from build123d import *

# Parameters (mm, degrees)
S01_RETAINING_FLANGE_R                         = 6.25
F_01_RETAINING_FLANGE_DEPTH                    = 0.4
F_02_START                                     = 0.4
S02_INNER_RACE_AND_SEALED_ROLLING_ASSE_R       = 6.05
F_02_INNER_RACE_AND_SEALED_ROLLING_ASSEM_DEPTH = 11
F_03_START                                     = 11.4
S03_MOUNTING_THRUST_FACE_R                     = 6.25
F_03_MOUNTING_THRUST_FACE_DEPTH                = 0.6
F_04_START                                     = 12
S04_SIX_MILLIMETRE_STUD_WITH_FINAL_8_M_R       = 3
F_04_SIX_MILLIMETRE_STUD_WITH_FINAL_8_MM_DEPTH = 16
F_05_START                                     = -0.1
S05_ASSEMBLY_DRIVE_SLOT_W                      = 8.4
S05_ASSEMBLY_DRIVE_SLOT_H                      = 1.4
F_05_ASSEMBLY_DRIVE_SLOT_DEPTH                 = 0.7


with BuildPart() as part:
    # S01 - Retaining flange → 01 - Retaining flange (new body)
    with BuildSketch(Plane.XY):
        Circle(S01_RETAINING_FLANGE_R)
    extrude(amount=F_01_RETAINING_FLANGE_DEPTH)

    # S02 - Inner race and sealed rolling assembly envelope → 02 - Inner race and sealed rolling assembly envelope (add)
    with BuildSketch(Plane.XY.offset(F_02_START)):
        Circle(S02_INNER_RACE_AND_SEALED_ROLLING_ASSE_R)
    extrude(amount=F_02_INNER_RACE_AND_SEALED_ROLLING_ASSEM_DEPTH)

    # S03 - Mounting thrust face → 03 - Mounting thrust face (add)
    with BuildSketch(Plane.XY.offset(F_03_START)):
        Circle(S03_MOUNTING_THRUST_FACE_R)
    extrude(amount=F_03_MOUNTING_THRUST_FACE_DEPTH)

    # S04 - Six millimetre stud with final 8 mm M6 thread envelope → 04 - Six millimetre stud with final 8 mm M6 thread envelope (add)
    with BuildSketch(Plane.XY.offset(F_04_START)):
        Circle(S04_SIX_MILLIMETRE_STUD_WITH_FINAL_8_M_R)
    extrude(amount=F_04_SIX_MILLIMETRE_STUD_WITH_FINAL_8_MM_DEPTH)

    # S05 - Assembly drive slot → 05 - Assembly drive slot (cut)
    with BuildSketch(Plane.XY.offset(F_05_START)):
        Rectangle(S05_ASSEMBLY_DRIVE_SLOT_W, S05_ASSEMBLY_DRIVE_SLOT_H)
    extrude(amount=F_05_ASSEMBLY_DRIVE_SLOT_DEPTH, mode=Mode.SUBTRACT)


solid = part.part
Could you check a few things on this model? Use its own coordinates, in mm. A direction names the side the tool comes from. Round coordinates to 2 decimals unless told otherwise and drop trailing zeros. Write each loop counter-clockwise with the first axis right and the second up, starting at its lowest first coordinate (ties: lowest second). Pieces come first, ordered by that corner, then holes. Notation, with made-up numbers: (12, 61) - (69, 61) arc R31 cw to (69, 87) - close; hole circle Ø11 at (68.5, 40). An arc over 180 degrees is marked (long way). Use a Markdown table: item, result.
Q1. For faces 1 (the cylindrical face through (5.96, 1.88, 0.2)), 2 (the flat face through (-1, -3, 12)), which set-ups out of +Z, -Z, +X, -X, +Y, -Y let a thin tool reach every point of the face, with its end or its side?
Output values:
| item | result |
|---|---|
| face 1 | +Z, -Z |
| face 2 | +Z |
Q2. Please list where these lines run through material, in increasing order: L1, parallel to Z at x = 1.75, y = 5.75; L2, parallel to X at y = -0.25, z = 6.5; L3, parallel to Y at x = 2.75, z = 10.75.
Output values:
| item | result |
|---|---|
| L1 | 0 to 12 |
| L2 | -6.04 to 6.04 |
| L3 | -5.39 to 5.39 |
Q3. Thinking about a two-plate mould opening in Y: for faces 3 (the cylindrical face through (5.589, -2.317, 5.823)), 4 (the flat face through (0, -1, 0)), 5 (the flat face through (0, 0, 0.6)), which applies, released by +Y, released by -Y, zero draft, split by the parting line, or undercut?
Output values:
| item | result |
|---|---|
| face 3 | split by the parting line |
| face 4 | zero draft |
| face 5 | undercut |
Q4. I want a section at A-A (x = 0). List the corners of the cut face in (y, z) for me.
Output values:
| item | result |
|---|---|
| outline | (-6.25, 0) - (-0.7, 0) - (-0.7, 0.6) - (0.7, 0.6) - (0.7, 0) - (6.25, 0) - (6.25, 0.4) - (6.05, 0.4) - (6.05, 11.4) - (6.25, 11.4) - (6.25, 12) - (3, 12) - (3, 28) - (-3, 28) - (-3, 12) - (-6.25, 12) - (-6.25, 11.4) - (-6.05, 11.4) - (-6.05, 0.4) - (-6.25, 0.4) - close |
Q5. I want a section at C-C (z = 6.25). List the corners of the cut face in (x, y) for me, plus the area to 3 significant figures.
Output values:
| item | result |
|---|---|
| outline | circle Ø12.1 at (0, 0) |
| area | 115 mm2 |
Q6. I want a section at B-B (y = 0). List the corners of the cut face in (x, z) for me, plus the area to 3 significant figures.
Output values:
| item | result |
|---|---|
| outline | (-6.25, 0) - (-4.2, 0) - (-4.2, 0.6) - (4.2, 0.6) - (4.2, 0) - (6.25, 0) - (6.25, 0.4) - (6.05, 0.4) - (6.05, 11.4) - (6.25, 11.4) - (6.25, 12) - (3, 12) - (3, 28) - (-3, 28) - (-3, 12) - (-6.25, 12) - (-6.25, 11.4) - (-6.05, 11.4) - (-6.05, 0.4) - (-6.25, 0.4) - close |
| area | 237 mm2 |
Q7. For pin 1 (2 mm diameter, centred on y = -1.5, z = 9, fed in from +X); pin 2 (0.5 mm diameter, centred on x = 1.5, z = 0.5, fed in from +Y); pin 3 (0.7 mm diameter, centred on y = -0.5, z = 0, fed in from -X), each with a flat end and sliding along its axis, tell me the tip position at first contact or that it passes through.
Output values:
| item | result |
|---|---|
| pin 1 | x = 6.03 |
| pin 2 | y = 6.12 |
| pin 3 | x = -6.25 |
Q8. I want a section at D-D (y = -2.5). List the corners of the cut face in (x, z) for me.
Output values:
| item | result |
|---|---|
| outline | (-5.73, 0) - (5.73, 0) - (5.73, 0.4) - (5.51, 0.4) - (5.51, 11.4) - (5.73, 11.4) - (5.73, 12) - (1.66, 12) - (1.66, 28) - (-1.66, 28) - (-1.66, 12) - (-5.73, 12) - (-5.73, 11.4) - (-5.51, 11.4) - (-5.51, 0.4) - (-5.73, 0.4) - close |
